Part model, mm, in its own coordinate system. Face numbers are marked on the shaded views. A direction names the side the tool comes from. Round coordinates to 2 decimals unless told otherwise and drop trailing zeros. Write each loop counter-clockwise with the first axis right and the second up, starting at its lowest first coordinate (ties: lowest second). Pieces come first, ordered by that corner, then holes. Notation, with made-up numbers: (63.5, 10.5) -> (111.5, 10.5) arc R17 cw to (111.5, 20.5) -> close; hole circle Ø11 at (-0.75, -5). An arc over 180 degrees is marked (long way). Use CSV: the item, a comma, the result in double quotes. Start each with the question number.
(1) Saw through at B-B (x = -30.5). Give the cut face in (y, z).
(2) Drop flat-ended pins along their axis: pin 1 (0.6 mm diameter, centred on x = -80, y = 6, fed in from -Z); pin 2 (8 mm diameter, centred on x = -79.5, z = 4, fed in from +Y); pin 3 (5 mm diameter, centred on x = -65, y = 2, fed in from +Z). Give the stop position or say it passes through.
(3) Probe line 1 (X direction, y = 6.75, z = -12); line 2 (Y direction, x = -75, z = 8); line 3 (X direction, y = 1.5, z = -52). List the from-to ranges inside material, lowest first. Write a range as [from, to].
(4) Saw through at A-A (z = -18). Give the cut face in (x, y).
(5) Which spindle directions (+Z, -Z, +X, -X, +Y, -Y) get a long thin tool onto all of the face, cutting with end or side? Do the marked faces 4, 5 and 6. Say none if no direction does.
(6) Saw through at D-D (x = -58.5). Give the cut face in (y, z), plus the area to 3 significant figures.
(7) Two-plate mould, pull along X, no slides. Class the marked faces 1, 2 and 3: released by +X, released by -X, zero draft, split by the parting line, or undercut.
(8) Saw through at C-C (y = 5). Count the separate pieces of the cut face and the enclosed holes in it, plus the area to 3 significant figures.
Autodesk Inventor part; units mm, degrees
ref_plane "YZ Plane" through (0, 0, 0) normal (1, 0, 0) x (0, 1, 0)
ref_plane "XZ Plane" through (0, 0, 0) normal (0, 1, 0) x (-1, 0, 0)
ref_plane "XY Plane" through (0, 0, 0) normal (0, 0, 1) x (1, 0, 0)
sketch "Sketch1" plane through (0, 0, 0) normal (0, 1, 0) x (-1, 0, 0)
  line L0 (0, 0) -> (0, -50)
  line L1 (90, -50) -> (90, 0)
  line L2 (90, -25) -> (90, -70)
  line L3 (90, -25) -> (90, 20)
  line L4 (90, 20) -> (60, 20)
  line L5 (90, -70) -> (60, -70)
  line L6 (60, 20) -> (45, 20)
  line L7 (60, -70) -> (45, -70)
  line L8 (45, -70) -> (0, -50)
  line L9 (45, 20) -> (0, 0)
extrude "Extrusion1" add sketch "Sketch1" along normal blind 9
fillet "Fillet1" radius 30 2 edges at (-90, 4.5, 20) (-90, 4.5, -70)
sketch "Sketch2" plane through (0, 9, 0) normal (0, 1, 0) x (1, 0, 0)
  arc A0 (-90, 10) -> (-60, -20) centre (-60, 10) ccw
  line L0 (-90, 10) -> (-84, 10)
  line L1 (-90, 40) -> (-90, 10)
  line L2 (-90, 40) -> (-84, 40)
  line L3 (-84, 40) -> (-84, 10)
  line L4 (-45, -20) -> (0, 0)
  line L5 (-45, -20) -> (-22.6116, -10.0496)
  line L6 (-22.6116, -10.0496) -> (-36.3188, -16.1417)
  line L7 (-22.6116, -10.0496) -> (-8.9044, -3.9575)
  line L8 (-8.9044, -3.9575) -> (-11.3413, 1.5253)
  line L9 (-36.3188, -16.1417) -> (-38.7556, -10.6588)
  line L10 (-38.7556, -10.6588) -> (-11.3413, 1.5253)
  line L11 (0, 50) -> (-45, 70)
  line L12 (-45, 70) -> (-22.6116, 60.0496)
  line L13 (-22.6116, 60.0496) -> (-36.3188, 66.1417)
  line L14 (-36.3188, 66.1417) -> (-38.7556, 60.6588)
  line L15 (-22.5, 60) -> (-8.7928, 53.9079)
  line L16 (-8.7928, 53.9079) -> (-11.2297, 48.4251)
  line L17 (-11.2297, 48.4251) -> (-38.5472, 61.1277)
  dimension "d11" = 6
extrude "Extrusion2" cut sketch "Sketch2" against normal blind 9
fillet "Fillet2" radius 8 2 edges at (0, 4.5, 0) (0, 4.5, -50)
sketch "Sketch3" plane through (0, 9, 0) normal (0, 1, 0) x (1, 0, 0)
  line L0 (-84, 40) -> (-84, 10)
  line L1 (-81, 10) -> (-81, 40)
  line L2 (-81, 40) -> (-79, 40)
  line L3 (-79, 40) -> (-79, 10)
  line L4 (-79, 10) -> (-81, 10)
  line L5 (-36.3188, -16.1417) -> (-38.7556, -10.6588)
  line L6 (-39.974, -7.9174) -> (-12.5597, 4.2668)
  line L7 (-12.5597, 4.2668) -> (-13.372, 6.0944)
  line L8 (-13.372, 6.0944) -> (-40.7863, -6.0898)
  line L9 (-40.7863, -6.0898) -> (-39.974, -7.9174)
  line L10 (-38.5472, 61.1277) -> (-38.7617, 60.6665)
  line L11 (-11.2297, 48.4251) -> (-38.5472, 61.1277)
  line L12 (-39.8122, 58.4074) -> (-12.4946, 45.7048)
  line L13 (-12.4946, 45.7048) -> (-13.3379, 43.8912)
  line L14 (-13.3379, 43.8912) -> (-40.6555, 56.5938)
  line L15 (-40.6555, 56.5938) -> (-39.8122, 58.4074)
  point P0 (0, 0)
extrude "Extrusion3" cut sketch "Sketch3" against normal blind 9
sketch "Sketch4" plane through (0, 9, 0) normal (0, 1, 0) x (1, 0, 0)
  arc A0 (-90, 10) -> (-60, -20) centre (-60, 10) ccw
  line L0 (-60, 10) -> (-81.2132, -11.2132)
  line L1 (-60, 10) -> (-30, 10) construction
  arc A1 (-60, 70) -> (-90, 40) centre (-60, 40) ccw
  line L2 (-60, 40) -> (-78.753, 58.753)
  line L3 (-60, 40) -> (-33.4792, 40) construction
  line L4 (0, 5.199) -> (0, 44.801)
  line L5 (0, 25) -> (-14, 25)
  line L6 (-81.2132, -11.2132) -> (-71.3137, -1.3137)
  line L7 (-81.2132, 61.2132) -> (-71.3137, 51.3137)
  circle A2 centre (-71.3137, -1.3137) radius 3.5
  circle A3 centre (-71.3137, 51.3137) radius 3.5
  circle A4 centre (-14, 25) radius 3.5
  point P0 (0, 0)
  dimension "d38" = 7
  dimension "d39" = 7
  dimension "d40" = 7
extrude "Extrusion4" add sketch "Sketch4" along normal blind 9
sketch "Sketch5" plane through (0, 0, 0) normal (0, -1, 0) x (1, 0, 0)
  point P0 (0, 0)
properties part number "palm"
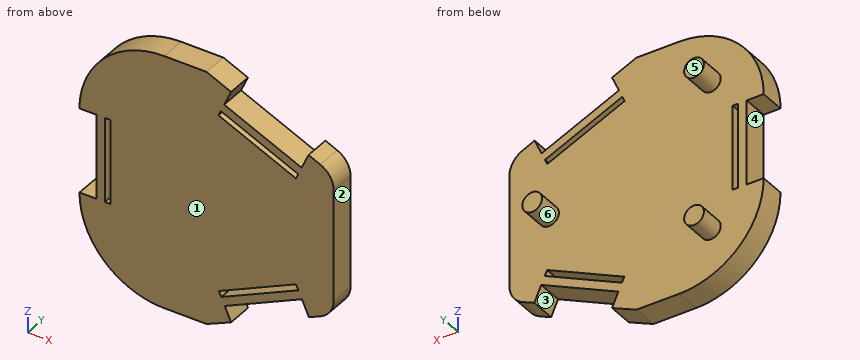
Answers:
1,outline,"(0, -57.39) -> (9, -57.39) -> (9, -54.08) -> (0, -54.08) -> close; (0, -51.87) -> (9, -51.87) -> (9, 1.52) -> (0, 1.52) -> close; (0, 3.71) -> (9, 3.71) -> (9, 6.99) -> (0, 6.99) -> close"
2,pin 1,"stops at z = -62.63"
2,pin 2,"stops at y = 9"
2,pin 3,"stops at z = 19.9"
3,line 1,"x = [-84, -81], [-79, 0]"
3,line 2,"y = [0, 9]"
3,line 3,"x = [-87.5, -30.78], [-26.03, -18.92], [-9.64, -4.51]"
4,outline,"(-84, 0) -> (-81, 0) -> (-81, 9) -> (-84, 9) -> close; (-79, 0) -> (0, 0) -> (0, 9) -> (-79, 9) -> close"
5,face 4,"-X, +Y, -Y"
5,face 5,"+Z, -Z, +X, -X, +Y"
5,face 6,"+Y"
6,outline,"(0, -70) -> (9, -70) -> (9, 20) -> (0, 20) -> close"
6,area,"810 mm²"
7,face 1,"zero draft"
7,face 2,"released by +X"
7,face 3,"undercut"
8,separate pieces,"1"
8,enclosed holes,"3"
8,area,"6,090 mm²"
